Design review of the part built by this model. Coordinates are the model's own, in mm. Face numbers are marked on the shaded views. A direction names the side the tool comes from. Give positions to 0.01 mm unless a question says otherwise; leave off trailing zeros. Loops run counter-clockwise (first coordinate to the right, second up) from the corner with the lowest first, then second, coordinate; pieces in that order, holes last. Notation, with made-up numbers: (-10, -2) - (1, -2) arc R15 ccw to (1, 22) - close; hole circle Ø5 at (-35.5, -12.75). An arc over 180 degrees is marked (long way). Write each question's results on one line, items separated by ' | '.
from build123d import *

# Parameters (mm, degrees)
F0_R     = 15.875
F1_DEPTH = 25.4


with BuildPart() as f1:
    # F0 (on Top) → F1 (new body)
    with BuildSketch(Plane.XY):
        with BuildLine():
            Line((-93.816891, -38.1), (58.583109, -38.1))
            ThreePointArc((58.583109, -38.1), (96.683109, 0), (58.583109, 38.1))
            Line((58.583109, 38.1), (7.783109, 38.1))
            Line((7.783109, 38.1), (7.783109, 25.4))
            Line((7.783109, 25.4), (-43.016891, 25.4))
            Line((-43.016891, 25.4), (-43.016891, 38.1))
            Line((-43.016891, 38.1), (-93.816891, 38.1))
            ThreePointArc((-93.816891, 38.1), (-131.916891, 0), (-93.816891, -38.1))
        make_face()
        with Locations((-93.816891, 0)):
            Circle(F0_R, mode=Mode.SUBTRACT)
        with Locations((58.583109, 0)):
            Circle(F0_R, mode=Mode.SUBTRACT)
    extrude(amount=F1_DEPTH)


solid = f1.part
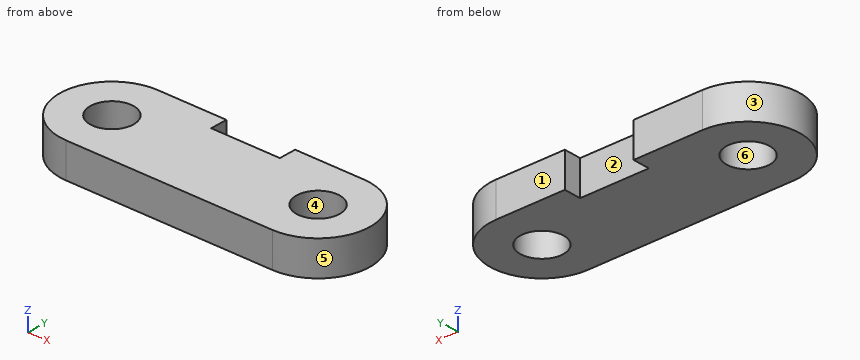
(1) Insertion check: P1, Ø6, axis at y = 14.5, z = 6.5, coming from the -X side; P2, Ø10, axis at y = 32, z = 17.5, coming from the +X side; P3, Ø3, axis at y = 23.5, z = 21, coming from the +X side; P4, Ø12, axis at x = 5, y = 27.5, coming from the -Z side. Each pin has a flat end and moves straight along its axis. Give the tip position at first contact, or say it passes through.
Answers below:
P1: x = -130.14 | P2: x = 85.46 | P3: x = 89.69 | P4: z = 0
(2) Wall thickness on line 1 along Y through (x, z) = (-99.5, 18); line 2 along X through (y, z) = (-7, 19.25); line 3 along X through (y, z) = (5, 5): over which ranges is each line inside the solid? List them lowest first. Write a range as from..to.
Answers below:
line 1: -37.67..-14.82, 14.82..37.67 | line 2: -131.27..-108.07, -79.57..44.33, 72.83..96.03 | line 3: -131.59..-108.88, -78.75..43.52, 73.65..96.35
(3) Take a section at D-D on x = -0.5. Give the boundary of the cut face in (y, z), plus the area to 3 significant figures.
Answers below:
outline: (-38.1, 0) - (25.4, 0) - (25.4, 25.4) - (-38.1, 25.4) - close | area: 1,610 mm2
(4) Take a section at B-B on z = 22. Give the boundary of the cut face in (x, y) (3 decimals), plus the area to 3 significant figures.
Answers below:
outline: (-93.817, -38.1) - (58.583, -38.1) arc R38.1 ccw to (58.583, 38.1) - (7.783, 38.1) - (7.783, 25.4) - (-43.017, 25.4) - (-43.017, 38.1) - (-93.817, 38.1) arc R38.1 ccw to start; hole circle Ø31.75 at (-93.817, 0); hole circle Ø31.75 at (58.583, 0) | area: 13,900 mm2
(5) Take a section at C-C on y = 30. Give the boundary of the cut face in (x, z).
Answers below:
outline: (-117.3, 0) - (-43.02, 0) - (-43.02, 25.4) - (-117.3, 25.4) - close; (7.78, 0) - (82.07, 0) - (82.07, 25.4) - (7.78, 25.4) - close
(6) Draft analysis for pull direction X (two halves, no side actions). For the marked faces 3, 4, 5 and 6, state which applies: pulls with the +X half, pulls with the -X half, needs draft (parallel to the pull), parting line crosses it, or undercut.
Answers below:
face 3: pulls with the -X half | face 4: undercut | face 5: pulls with the +X half | face 6: undercut
(7) Tool access review of the marked faces 1 and 2: name each direction out of +Z, -Z, +X, -X, +Y, -Y from which nothing blocks a thin tool from reaching the whole face with its end or side.
Answers below:
face 1: +Z, -Z, +X, -X, +Y | face 2: +Z, -Z, +Y
(8) Take a section at A-A on y = 0. Give the boundary of the cut face in (x, z), plus the area to 3 significant figures.
Answers below:
outline: (-131.92, 0) - (-109.69, 0) - (-109.69, 25.4) - (-131.92, 25.4) - close; (-77.94, 0) - (42.71, 0) - (42.71, 25.4) - (-77.94, 25.4) - close; (74.46, 0) - (96.68, 0) - (96.68, 25.4) - (74.46, 25.4) - close | area: 4,190 mm2
